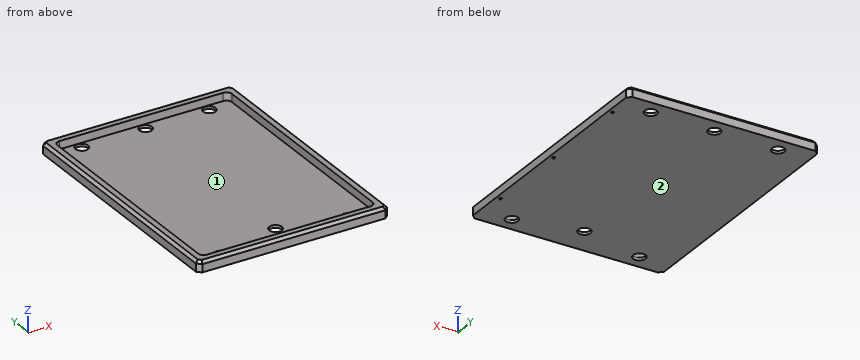
```python
from build123d import *

# Parameters (mm, degrees)
SKETCH1_W                 = 228.6
SKETCH1_H                 = 304.8
BOSS_EXTRUDE1_DEPTH       = 12.7
CUT_EXTRUDE1_DEPTH        = 9.525
SKETCH4_R                 = 7.5
CUT_EXTRUDE2_DEPTH        = 4.175
M4X0_7_TAPPED_HOLE1_D     = 3.3
M4X0_7_TAPPED_HOLE1_DEPTH = 8
M4X0_7_TAPPED_HOLE1_TIP   = 0.991420021
CHAMFER1_SIZE             = 4.7625
CHAMFER2_SIZE             = 3.175


with BuildPart() as part:
    # Sketch1 → Boss-Extrude1 (new body)
    with BuildSketch(Plane.XY):
        Rectangle(SKETCH1_W, SKETCH1_H)
    extrude(amount=BOSS_EXTRUDE1_DEPTH)

    # Sketch2 → Cut-Extrude1 (cut)
    with BuildSketch(Plane.XY.offset(12.7)):
        with BuildLine():
            Line((97.95, -142.4), (-97.95, -142.4))
            ThreePointArc((-97.95, -142.4), (-102.440128061, -140.540128061), (-104.3, -136.05))
            Line((-104.3, -136.05), (-104.3, 136.05))
            ThreePointArc((-104.3, 136.05), (-102.440128061, 140.540128061), (-97.95, 142.4))
            Line((-97.95, 142.4), (97.95, 142.4))
            ThreePointArc((97.95, 142.4), (102.440128061, 140.540128061), (104.3, 136.05))
            Line((104.3, 136.05), (104.3, -136.05))
            ThreePointArc((104.3, -136.05), (102.440128061, -140.540128061), (97.95, -142.4))
        make_face()
    extrude(amount=-CUT_EXTRUDE1_DEPTH, mode=Mode.SUBTRACT)

    # Sketch4 → Cut-Extrude2 (cut, through all)
    with BuildSketch(Plane.XY.offset(3.175)):
        with Locations((-76.2, 134.05)):
            Circle(SKETCH4_R)
        with Locations((76.2, 134.05)):
            Circle(SKETCH4_R)
        with Locations((-76.2, -134.05)):
            Circle(SKETCH4_R)
        with Locations((76.2, -134.05)):
            Circle(SKETCH4_R)
        with Locations((0, 134.05)):
            Circle(SKETCH4_R)
        with Locations((0, -117)):
            Circle(SKETCH4_R)
    extrude(amount=-CUT_EXTRUDE2_DEPTH, mode=Mode.SUBTRACT)

    # M4x0.7 Tapped Hole1
    with Locations(Plane(origin=(0, 0, 0), x_dir=(-1, 0, 0), z_dir=(0, 0, -1))):
        with Locations((-109.3, -102.4), (-109.3, 0), (-109.3, 113.6)):
            Hole(M4X0_7_TAPPED_HOLE1_D / 2, depth=M4X0_7_TAPPED_HOLE1_DEPTH)
            with Locations((0, 0, -(M4X0_7_TAPPED_HOLE1_DEPTH + M4X0_7_TAPPED_HOLE1_TIP / 2))):  # 118° drill point
                Cone(0, M4X0_7_TAPPED_HOLE1_D / 2, M4X0_7_TAPPED_HOLE1_TIP, mode=Mode.SUBTRACT)

    # Chamfer1
    chamfer1_edges = [part.edges().sort_by_distance(p)[0] for p in [
        (-114.3, 152.4, 6.35),
        (114.3, 152.4, 6.35),
        (114.3, -152.4, 6.35),
        (-114.3, -152.4, 6.35),
    ]]
    chamfer(chamfer1_edges, length=CHAMFER1_SIZE)

    # Chamfer2
    chamfer2_edges = [part.edges().sort_by_distance(p)[0] for p in [
        (0, -152.4, 12.7),
        (-114.3, 0, 12.7),
        (114.3, 0, 12.7),
        (0, 152.4, 12.7),
        (111.91875, 150.01875, 12.7),
        (-111.91875, 150.01875, 12.7),
        (111.91875, -150.01875, 12.7),
        (-111.91875, -150.01875, 12.7),
    ]]
    chamfer(chamfer2_edges, length=CHAMFER2_SIZE)


solid = part.part
```
Source: CAD feature listing. Evaluate the final solid. Frame: model axes, mm. Face numbers are marked on the shaded views. Give positions to 0.01 mm unless a question says otherwise; leave off trailing zeros. Loops run counter-clockwise (first coordinate to the right, second up) from the corner with the lowest first, then second, coordinate; pieces in that order, holes last. Notation, with made-up numbers: (51.5, 43.5) - (95.5, 43.5) arc R14 cw to (95.5, 47.5) - close; hole circle Ø8 at (45.25, 29.25). An arc over 180 degrees is marked (long way). Use CSV: the item, a comma, the result in double quotes. Start each with the question number.
1. Ray query, L1, parallel to Y at x = 109.3, z = 3; L2, parallel to Y at x = 76.2, z = 1.45; L3, parallel to X at y = -123, z = 3.25. Return the intervals inside material, ascending.
2. Section C-C (x = -49.5). Output: boundary loops of the cut face in (y, z) (3 decimals).
3. Section B-B (y = -32). Output: boundary loops of the cut face in (x, z) (3 decimals), then the cut area to 3 significant figures.
4. Draft query along Y for the marked faces 1 and 2. Return one class per face: +Y half, -Y half, draft (parallel to the pull), parting line (faces both ways), or undercut.
5. Pin query (flat end, axial travel): pin 1 (12 mm diameter, centred on x = 76.2, y = -134.05, fed in from -Z); pin 2 (2.5 mm diameter, centred on x = 109.3, y = 113.6, fed in from -Z). Return the tip coordinate at first contact, or that it passes through.
6. Section A-A (x = 0). Output: boundary loops of the cut face in (y, z) (3 decimals).
Response:
1,L1,"-152.4 to -104.05, -100.75 to -1.65, 1.65 to 111.95, 115.25 to 152.4"
1,L2,"-152.4 to -141.55, -126.55 to 126.55, 141.55 to 152.4"
1,L3,"-114.3 to -104.3, 104.3 to 114.3"
2,outline,"(-152.4, 0) - (152.4, 0) - (152.4, 9.525) - (149.225, 12.7) - (142.4, 12.7) - (142.4, 3.175) - (-142.4, 3.175) - (-142.4, 12.7) - (-149.225, 12.7) - (-152.4, 9.525) - close"
3,outline,"(-114.3, 0) - (114.3, 0) - (114.3, 9.525) - (111.125, 12.7) - (104.3, 12.7) - (104.3, 3.175) - (-104.3, 3.175) - (-104.3, 12.7) - (-111.125, 12.7) - (-114.3, 9.525) - close"
3,area,"906 mm²"
4,face 1,"undercut"
4,face 2,"draft"
5,pin 1,"through"
5,pin 2,"z = 8.24"
6,outline,"(-152.4, 0) - (-124.5, 0) - (-124.5, 3.175) - (-142.4, 3.175) - (-142.4, 12.7) - (-149.225, 12.7) - (-152.4, 9.525) - close; (-109.5, 0) - (126.55, 0) - (126.55, 3.175) - (-109.5, 3.175) - close; (141.55, 0) - (152.4, 0) - (152.4, 9.525) - (149.225, 12.7) - (142.4, 12.7) - (142.4, 3.175) - (141.55, 3.175) - close"
